```python
from build123d import *

# Parameters (mm, degrees)
SKETCH1_R           = 1.375
BOSS_EXTRUDE1_DEPTH = 4


with BuildPart() as part:
    # Sketch1 → Boss-Extrude1 (new body)
    with BuildSketch(Plane(origin=(0, 0, 0), x_dir=(1, 0, 0), z_dir=(0, 1, 0))):
        with BuildLine():
            Line((55, 0), (280, 0))
            ThreePointArc((280, 0), (318.890872965, 16.109127035), (335, 55))
            Line((335, 55), (335, 71))
            Line((335, 71), (313.5, 71))
            Line((313.5, 71), (313.5, 75.5))
            ThreePointArc((313.5, 75.5), (310.5, 78.5), (307.5, 75.5))
            Line((307.5, 75.5), (307.5, 71))
            Line((307.5, 71), (255.5, 71))
            Line((255.5, 71), (255.5, 75.5))
            ThreePointArc((255.5, 75.5), (254.621320344, 77.621320344), (252.5, 78.5))
            Line((252.5, 78.5), (248, 78.5))
            Line((248, 78.5), (248, 91))
            Line((248, 91), (238, 91))
            Line((238, 91), (238, 109))
            Line((238, 109), (248, 109))
            Line((248, 109), (248, 121.5))
            Line((248, 121.5), (252.5, 121.5))
            ThreePointArc((252.5, 121.5), (254.621320344, 122.378679656), (255.5, 124.5))
            Line((255.5, 124.5), (255.5, 129))
            Line((255.5, 129), (307.5, 129))
            Line((307.5, 129), (307.5, 124.5))
            ThreePointArc((307.5, 124.5), (310.5, 121.5), (313.5, 124.5))
            Line((313.5, 124.5), (313.5, 129))
            Line((313.5, 129), (335, 129))
            Line((335, 129), (335, 145))
            ThreePointArc((335, 145), (318.890872965, 183.890872965), (280, 200))
            Line((280, 200), (55, 200))
            ThreePointArc((55, 200), (16.109127035, 183.890872965), (0, 145))
            Line((0, 145), (0, 55))
            ThreePointArc((0, 55), (16.109127035, 16.109127035), (55, 0))
        make_face()
        with Locations(Location((252.5, 124.5, 0), (0, 0, 270))):
            Circle(SKETCH1_R, mode=Mode.SUBTRACT)
        with Locations(Location((252.5, 75.5, 0), (0, 0, 90))):
            Circle(SKETCH1_R, mode=Mode.SUBTRACT)
        with Locations(Location((310.5, 124.5, 0), (0, 0, 270))):
            Circle(SKETCH1_R, mode=Mode.SUBTRACT)
        with Locations(Location((310.5, 75.5, 0), (0, 0, 90))):
            Circle(SKETCH1_R, mode=Mode.SUBTRACT)
        with BuildLine():
            Line((55, 25), (280, 25))
            ThreePointArc((280, 25), (297.748239349, 30.813226755), (308.618176043, 46))
            Line((308.618176043, 46), (223, 46))
            Line((223, 46), (223, 154))
            Line((223, 154), (308.618176043, 154))
            ThreePointArc((308.618176043, 154), (297.748239349, 169.186773245), (280, 175))
            Line((280, 175), (55, 175))
            ThreePointArc((55, 175), (33.786796564, 166.213203436), (25, 145))
            Line((25, 145), (25, 55))
            ThreePointArc((25, 55), (33.786796564, 33.786796564), (55, 25))
        make_face(mode=Mode.SUBTRACT)
    extrude(amount=BOSS_EXTRUDE1_DEPTH)


solid = part.part
```
Here's how the part is built. I have some questions about the finished solid (model axes, mm). A direction names the side the tool comes from. Give positions to 0.01 mm unless a question says otherwise; leave off trailing zeros. Write each loop counter-clockwise with the first axis right and the second up, starting at its lowest first coordinate (ties: lowest second). Pieces come first, ordered by that corner, then holes.
(1) Imagine slicing it at C-C, the plane x = 266. Write out the boundary of the cut face in (y, z), and give its area (3 significant figures).
Output values:
outline: (0, -200) - (4, -200) - (4, -175) - (0, -175) - close; (0, -154) - (4, -154) - (4, -129) - (0, -129) - close; (0, -71) - (4, -71) - (4, -46) - (0, -46) - close; (0, -25) - (4, -25) - (4, 0) - (0, 0) - close
area: 400 mm2
(2) Thinking about a two-plate mould opening in Z: for faces 1 (the face through (33.555, 1.972, -34.021)), 2 (the face through (319.316, 1.972, -183.461)), 3 (the face through (240, 4, -79)), which applies, pulls with the +Z half, pulls with the -Z half, needs draft (parallel to the pull), parting line crosses it, or undercut?
Output values:
face 1: undercut
face 2: pulls with the -Z half
face 3: needs draft
(3) Imagine slicing it at D-D, the plane y = 2.8. Count the separate pieces of the cut face and the enclosed holes in it, and give its area (3 significant figures).
Output values:
separate pieces: 1
enclosed holes: 5
area: 26,800 mm2
(4) Will these pins go through, and if not, where does the flat tip stop? pin 1 (2 mm diameter, centred on y = 1.5, z = -89, fed in from +X); pin 2 (2 mm diameter, centred on y = 2.5, z = -101.5, fed in from +X); pin 3 (2 mm diameter, centred on x = 252.5, z = -75.5, fed in from +Y); pin 4 (1.2 mm diameter, centred on y = 2.5, z = -73, fed in from +X).
Output values:
pin 1: stops at x = 248
pin 2: stops at x = 238
pin 3: passes through
pin 4: stops at x = 313.5
(5) Imagine slicing it at B-B, the plane x = 112.5. Write out the boundary of the cut face in (y, z), and give its area (3 significant figures).
Output values:
outline: (0, -200) - (4, -200) - (4, -175) - (0, -175) - close; (0, -25) - (4, -25) - (4, 0) - (0, 0) - close
area: 200 mm2
(6) If I drill on L1, parallel to X at y = 1.1, z = -124.5 (3 decimals); L2, parallel to Z at x = 252.5, y = 1 (3 decimals); L3, parallel to Z at x = 275.5, y = 3.3, over which ranges is the centre line in solid material (lowest first)?
Output values:
L1: x = 0 to 25, 223 to 251.125, 253.875 to 255.5, 307.5 to 309.125, 311.875 to 313.5
L2: z = -200 to -175, -154 to -125.875, -123.125 to -121.5, -78.5 to -76.875, -74.125 to -46, -25 to 0
L3: z = -200 to -175, -154 to -129, -71 to -46, -25 to 0
(7) On a 3-axis mill with a long thin cutter (end or side, diameter ignored), from which of +Z, -Z, +X, -X, +Y, -Y can I reach the whole of each face in a straight line? I mean faces 4 (the face through (16.539, 1.972, -184.316)), 5 (the face through (34.021, 1.972, -166.445)). Say none if no direction works.
Output values:
face 4: -Z, -X, +Y, -Y
face 5: +Y, -Y
(8) Imagine slicing it at A-A, the plane z = -87. Write out the boundary of the cut face in (x, y).
Output values:
outline: (0, 0) - (25, 0) - (25, 4) - (0, 4) - close; (223, 0) - (248, 0) - (248, 4) - (223, 4) - close
